Geometry check sheet. Reference: the model listing, model coordinates, mm. A direction names the side the tool comes from. Round coordinates to 2 decimals unless told otherwise and drop trailing zeros. Write each loop counter-clockwise with the first axis right and the second up, starting at its lowest first coordinate (ties: lowest second). Pieces come first, ordered by that corner, then holes. Notation, with made-up numbers: M 14,49.5 L 24,49.5 A34 ccw 24,83.5 Z; hole C -14,-16 d4. An arc over 180 degrees is marked long. Answer in a Markdown table with one row per item. Add a question column.
from build123d import *

# Parameters (mm, degrees)
F0_R     = 17.6630626633
F1_DEPTH = 55.1
F2_R     = 5
F3_R     = 6.360255015
F4_DEPTH = 4.4
F5_DEPTH = 9.1
F6_DEPTH = 6.2
F8_DEPTH = 0.8
F9_R     = 2.1727922061
F10_R    = 1.9313708499


# Not quite as in the source:
# - the program builds the solid bodies; features that only make, move or delete a surface that nothing else refers to are left out


with BuildPart() as f1:
    # F0 (on Top) → F1 (new body)
    with BuildSketch(Plane.XY):
        with Locations((-60.169108212, 0)):
            Circle(F0_R)
    extrude(amount=F1_DEPTH)

    # F2
    f2_edges = [f1.edges().sort_by_distance(p)[0] for p in [
        (-77.832171, 0, 0),
        (-77.832171, 0, 55.1),
    ]]
    fillet(f2_edges, radius=F2_R)

    # F3 (on face) → F4 (join)
    with BuildSketch(Plane.XY.offset(55.1)):
        with Locations((-59.8526485264, -4.0257023647)):
            Circle(F3_R)
    extrude(amount=F4_DEPTH)

    # F5 (cut): a face of the model
    f5_faces = [f1.faces().sort_by_distance(p)[0] for p in [
        (-59.8526485264, -4.0257023647, 59.5),
    ]]
    extrude(f5_faces, amount=-F5_DEPTH, mode=Mode.SUBTRACT)

    # F6 (cut): a face of the model
    f6_faces = [f1.faces().sort_by_distance(p)[0] for p in [
        (-59.8526485264, -4.0257023647, 50.4),
    ]]
    extrude(f6_faces, amount=-F6_DEPTH, mode=Mode.SUBTRACT)

    # F7 (on face) → F8 (join)
    with BuildSketch(Plane.XY.offset(55.1)):
        with BuildLine():
            Line((-53.6922231234, 9.6299564466), (-65.4776543379, 9.6299564466))
            Line((-65.4776543379, 9.6299564466), (-65.4776543379, -1.0571752086))
            ThreePointArc((-65.4776543379, -1.0571752086), (-59.1093847847, 2.2909742033), (-53.6922231234, -2.4439303493))
            Line((-53.6922231234, -2.4439303493), (-53.6922231234, 9.6299564466))
        make_face()
    extrude(amount=F8_DEPTH)

    # F9
    f9_edges = [f1.edges().sort_by_distance(p)[0] for p in [
        (-53.692223, 9.629956, 55.5),
    ]]
    fillet(f9_edges, radius=F9_R)

    # F10
    f10_edges = [f1.edges().sort_by_distance(p)[0] for p in [
        (-65.477654, 9.629956, 55.5),
    ]]
    fillet(f10_edges, radius=F10_R)


solid = f1.part
Item 1: Section check B-B, the plane z = 32.5. Record the boundary of the cut face in (x, y).
Item 2: Gauge pin test, flat ends, axial feed: pin 1 Ø3 at (x, z) = (-64, 27) entering from +Y; pin 2 Ø1 at (y, z) = (-1.5, 27) entering from -X; pin 3 Ø5 at (x, z) = (-73, 26.5) entering from +Y. Record the tip position at first contact, or that the pin passes through.
Item 3: Access from +Z, -Z, +X, -X, +Y, -Y to the whole of each face (thin tool, end or side, straight path). Record for faces 4 (the cylindrical face through (-64.897, 9.079, 55.506)), 5 (the flat face through (-60, 0, 0)).
Item 4: Mould release check, pull along X, two halves, no side actions. Record for faces 1 (the cylindrical face through (-54.312, 8.977, 55.506)), 2 (the cylindrical face through (-77.815, 0.777, 27.234)), 3 (the flat face through (-60, -4, 44.2)): +X half, -X half, draft (parallel to the pull), parting line (faces both ways), or undercut.
Item 5: Section check C-C, the plane z = 52. Record the boundary of the cut face in (x, y).
Item 6: Scan lines: probe 1 along Z at (x, y) = (-59, -10); probe 2 along Z at (x, y) = (-65.5, 8); probe 3 along X at (y, z) = (-8, 45.5). Record each from-to range of solid material in increasing order. Write a range as from..to.
Item 7: Section check A-A, the plane y = 0. Record the boundary of the cut face in (x, z).
Result sheet:
| question | item | result |
|---|---|---|
| 1 | outline | C -60.17,0 d35.33 |
| 2 | pin 1 | stops at y = 17.51 |
| 2 | pin 2 | stops at x = -77.8 |
| 2 | pin 3 | stops at y = 14.33 |
| 3 | face 4 | +Z, -X, +Y |
| 3 | face 5 | -Z, +X, -X, +Y, -Y |
| 4 | face 1 | +X half |
| 4 | face 2 | parting line |
| 4 | face 3 | undercut |
| 5 | outline | C -60.17,0 d34.58; hole C -59.85,-4.03 d12.72 |
| 6 | probe 1 | z = 0..44.2 |
| 6 | probe 2 | z = 0..55.1 |
| 6 | probe 3 | x = -75.92..-64.82, -54.89..-44.42 |
| 7 | outline | M -77.83,5 A5 ccw -72.83,0 L -47.51,0 A5 ccw -42.51,5 L -42.51,50.1 A5 ccw -47.51,55.1 L -53.69,55.1 L -53.69,55.9 L -54.93,55.9 L -54.93,44.2 L -64.78,44.2 L -64.78,55.9 L -65.48,55.9 L -65.48,55.1 L -72.83,55.1 A5 ccw -77.83,50.1 Z |
